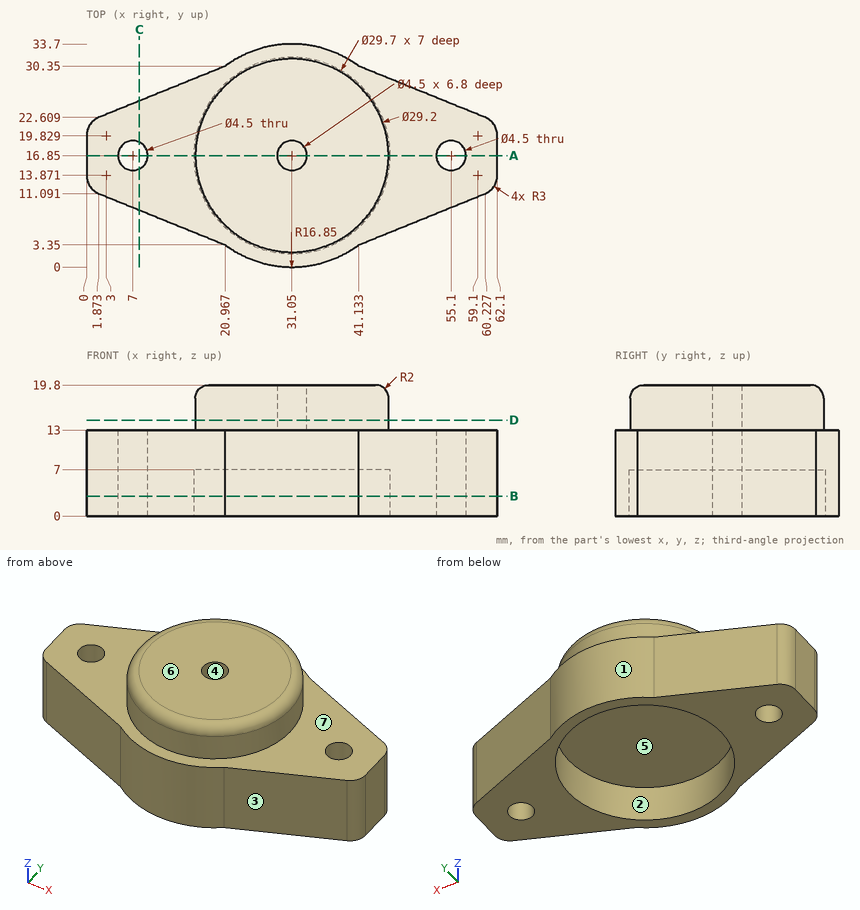
The figure shows three views and two pictorial views of one solid part (mm, origin at its lowest corner). Answer the questions. A direction names the side the tool comes from. Give positions to 0.01 mm unless a question says otherwise; leave off trailing zeros. Order: outer loops, then holes, each group sorted by start corner. A loop starts at its lowest first (then second) coordinate and runs counter-clockwise, first axis right, second up. Notation, with made-up numbers: (66, 34.5) -> (75, 34.5) arc R32 cw to (75, 60.5) -> close; hole circle Ø7 at (1, 30). An arc over 180 degrees is marked (long way). Answer as CSV lines item,"result". Start each with the question number.
(1) Section D-D, the plane z = 14.5 is taken. Write down the section's boundary in (x, y), plus the area to 3 significant figures.
(2) Each of these flat-tipped pins is pushed along its axis until it touches: pin 1 Ø4 at (y, z) = (25.5, 13) entering from +X; pin 2 Ø5 at (y, z) = (25.5, 16) entering from -X; pin 3 Ø1.5 at (y, z) = (28.5, 7.5) entering from +X (1 decimal). Where does it stop, or does it pass through?
(3) For a pull along Y with two mould halves and no side action, classify the marked faces 1, 2, 3 and 4 as released by +Y, released by -Y, zero draft, split by the parting line, or undercut.
(4) Consider line 1 along Y through (x, z) = (30.5, 6.5); line 2 along X through (y, z) = (18.5, 11.25); line 3 along Z through (x, y) = (3, 20.5). Determine where each line is inside the solid, lowest interval first.
(5) Section C-C, the plane x = 8 is taken. Write down the section's boundary in (y, z) (1 decimal), plus the area to 3 significant figures.
(6) Which of the six approach directions +Z, -Z, +X, -X, +Y, -Y give full straight-line access (tool end or side, diameter ignored) to the marked faces 5, 6 and 7?
(7) Section B-B, the plane z = 3 is taken. Write down the section's boundary in (x, y).
(8) Section A-A, the plane y = 16.85 is taken. Write down the section's boundary in (x, z), plus the area to 3 significant figures.
Entries:
1,outline,"circle Ø29.2 at (31.05, 16.85); hole circle Ø4.5 at (31.05, 16.85)"
1,area,"654 mm²"
2,pin 1,"x = 58.03"
2,pin 2,"x = 17.81"
2,pin 3,"x = 47.5"
3,face 1,"released by +Y"
3,face 2,"undercut"
3,face 3,"released by -Y"
3,face 4,"undercut"
4,line 1,"0.01 to 2.01, 31.69 to 33.69"
4,line 2,"0 to 5.47, 8.53 to 53.57, 56.63 to 62.1"
4,line 3,"0 to 13"
5,outline,"(8.6, 0) -> (14.8, 0) -> (14.8, 13) -> (8.6, 13) -> close; (18.9, 0) -> (25.1, 0) -> (25.1, 13) -> (18.9, 13) -> close"
5,area,"162 mm²"
6,face 5,"-Z"
6,face 6,"+Z, +X, -X, +Y, -Y"
6,face 7,"+Z"
7,outline,"(0, 13.87) arc R3 ccw to (1.87, 11.09) -> (20.97, 3.35) arc R16.85 ccw to (41.13, 3.35) -> (60.23, 11.09) arc R3 ccw to (62.1, 13.87) -> (62.1, 19.83) arc R3 ccw to (60.23, 22.61) -> (41.13, 30.35) arc R16.85 ccw to (20.97, 30.35) -> (1.87, 22.61) arc R3 ccw to (0, 19.83) -> close; hole circle Ø4.5 at (7, 16.85); hole circle Ø29.7 at (31.05, 16.85); hole circle Ø4.5 at (55.1, 16.85)"
8,outline,"(0, 0) -> (4.75, 0) -> (4.75, 13) -> (0, 13) -> close; (9.25, 0) -> (16.2, 0) -> (16.2, 7) -> (45.9, 7) -> (45.9, 0) -> (52.85, 0) -> (52.85, 13) -> (45.65, 13) -> (45.65, 17.8) arc R2 ccw to (43.65, 19.8) -> (33.3, 19.8) -> (33.3, 13) -> (28.8, 13) -> (28.8, 19.8) -> (18.45, 19.8) arc R2 ccw to (16.45, 17.8) -> (16.45, 13) -> (9.25, 13) -> close; (57.35, 0) -> (62.1, 0) -> (62.1, 13) -> (57.35, 13) -> close"
8,area,"649 mm²"
